Check sheet for the modelled part. Datum: model origin and axes. Units: mm. A direction names the side the tool comes from. Give positions to 0.01 mm unless a question says otherwise; leave off trailing zeros. Order: outer loops, then holes, each group sorted by start corner. A loop starts at its lowest first (then second) coordinate and runs counter-clockwise, first axis right, second up. Notation, with made-up numbers: M 11,32.5 L 28,32.5 A21 ccw 28,54.5 Z; hole C 2.5,49 d7. An arc over 180 degrees is marked long. Return JSON: item names as keys, results as strings. Group by question number.
from build123d import *

# Parameters (mm, degrees)
F0_W     = 401.32
F0_H     = 807.72
F1_DEPTH = 243.84
F2_R     = 60.96
F3_DEPTH = 45.72
F4_W     = 340.36
F4_H     = 746.76
F5_DEPTH = 218.44
F6_R     = 82.55
F7_DEPTH = 213.36
F8_R     = 60.96
F9_DEPTH = 203.2


with BuildPart() as f1:
    # F0 (on Top) → F1 (new body)
    with BuildSketch(Plane.XY):
        with Locations((32.376148, 375.04495)):
            Rectangle(F0_W, F0_H)
    extrude(amount=F1_DEPTH)

    # F2 (on face) → F3 (join)
    with BuildSketch(Plane.XY.offset(243.84)):
        with Locations((-69.223852, 70.24495)):
            Circle(F2_R)
        with Locations((-69.223852, 273.44495)):
            Circle(F2_R)
        with Locations((-69.223852, 476.64495)):
            Circle(F2_R)
        with Locations((-69.223852, 679.84495)):
            Circle(F2_R)
        with Locations((133.976148, 70.24495)):
            Circle(F2_R)
        with Locations((133.976148, 273.44495)):
            Circle(F2_R)
        with Locations((133.976148, 476.64495)):
            Circle(F2_R)
        with Locations((133.976148, 679.84495)):
            Circle(F2_R)
    extrude(amount=F3_DEPTH)

    # F4 (on face) → F5 (cut)
    with BuildSketch(Plane(origin=(0, 0, 0), x_dir=(1, 0, 0), z_dir=(0, 0, -1))):
        with Locations((32.376148, -375.04495)):
            Rectangle(F4_W, F4_H)
    extrude(amount=-F5_DEPTH, mode=Mode.SUBTRACT)

    # F6 (on face) → F7 (join)
    with BuildSketch(Plane(origin=(0, 0, 218.44), x_dir=(1, 0, 0), z_dir=(0, 0, -1))):
        with Locations((32.376148, -578.24495)):
            Circle(F6_R)
        with Locations((32.376148, -375.04495)):
            Circle(F6_R)
        with Locations((32.376148, -171.84495)):
            Circle(F6_R)
    extrude(amount=F7_DEPTH)

    # F8 (on face) → F9 (cut)
    with BuildSketch(Plane(origin=(0, 0, 5.08), x_dir=(1, 0, 0), z_dir=(0, 0, -1))):
        with Locations((32.376148, -171.84495)):
            Circle(F8_R)
        with Locations((32.376148, -375.04495)):
            Circle(F8_R)
        with Locations((32.376148, -578.24495)):
            Circle(F8_R)
    extrude(amount=-F9_DEPTH, mode=Mode.SUBTRACT)


solid = f1.part
1) Release check for a two-part mould opening along X. For faces 4 (the face through (233.036, 369, 120)), 5 (the face through (133, 477, 289.56)), 6 (the face through (120.761, 10.735, 266.38)) record: released by +X, released by -X, zero draft, split by the parting line, or undercut.
2) Depth check by flat-ended pin: P1, Ø10, axis at x = -58, y = 346.5, coming from the -Z side; P2, Ø1, axis at x = -4.5, y = 107.5, coming from the -Z side. Enter the tip coordinate at first touch or a pass-through.
3) Tool access check on faces 1 (the face through (-70, 681, 289.56)), 2 (the face through (30, 381, 243.84)), 3 (the face through (25.88, 639.01, 5.08)). Record the directions out of +Z, -Z, +X, -X, +Y, -Y that give a thin tool (end or side, any length) a straight path to the whole face; none if there is none.
4) Sectioned sample at C-C on y = 359. Record the boundary of the cut face in (x, z), then the cut area to 3 significant figures.
5) Material ranges on line 1 along Y through (x, z) = (130.5, 248); line 2 along Y through (x, z) = (157, 155); line 3 along X through (y, z) = (410, 38), recorded low to high.
6) Sectioned sample at B-B on x = 147.5. Record the boundary of the cut face in (y, z).
7) Sectioned sample at A-A on z = 195. Record the boundary of the cut face in (x, y).
Reply:
{
 "1": {"face 4": "released by +X", "face 5": "zero draft", "face 6": "undercut"},
 "2": {"P1": "z = 218.44", "P2": "z = 5.08"},
 "3": {"face 1": "+Z, +X, -X, +Y, -Y", "face 2": "+Z", "face 3": "-Z"},
 "4": {"outline": "M -168.28,0 L -137.8,0 L -137.8,218.44 L -48.6,218.44 L -48.6,5.08 L -26.43,5.08 L -26.43,208.28 L 91.19,208.28 L 91.19,5.08 L 113.35,5.08 L 113.35,218.44 L 202.56,218.44 L 202.56,0 L 233.04,0 L 233.04,243.84 L -168.28,243.84 Z", "area": "34,200 mm^2"},
 "5": {"line 1": "9.38 to 131.11, 212.58 to 334.31, 415.78 to 537.51, 618.98 to 740.71", "line 2": "-28.82 to 1.66, 748.42 to 778.9", "line 3": "-168.28 to -137.8, -42.41 to -17.57, 82.32 to 107.16, 202.56 to 233.04"},
 "6": {"outline": "M -28.82,0 L 1.66,0 L 1.66,218.44 L 748.42,218.44 L 748.42,0 L 778.9,0 L 778.9,243.84 L 739.29,243.84 L 739.29,289.56 L 620.4,289.56 L 620.4,243.84 L 536.09,243.84 L 536.09,289.56 L 417.2,289.56 L 417.2,243.84 L 332.89,243.84 L 332.89,289.56 L 214,289.56 L 214,243.84 L 129.69,243.84 L 129.69,289.56 L 10.8,289.56 L 10.8,243.84 L -28.82,243.84 Z"},
 "7": {"outline": "M -168.28,-28.82 L 233.04,-28.82 L 233.04,778.9 L -168.28,778.9 Z; C 32.38,171.84 d165.1; C 32.38,375.04 d165.1; C 32.38,578.24 d165.1; hole M -137.8,1.66 L 202.56,1.66 L 202.56,748.42 L -137.8,748.42 Z; hole C 32.38,171.84 d121.92; hole C 32.38,375.04 d121.92; hole C 32.38,578.24 d121.92"}
}
